Source: CAD feature listing. Evaluate the final solid. Frame: model axes, mm. Give positions to 0.01 mm unless a question says otherwise; leave off trailing zeros. Return JSON: item names as keys, results as strings.
from build123d import *

# Parameters (mm, degrees)
SWEEP1_PROFILE_R     = 13.49375
CUT_SWEEP1_PROFILE_R = 9.525


with BuildPart() as part:
    # Sweep1: sweep along a curve in space
    with BuildLine() as sweep1_path:
        Line((1.507056985, -46.735868675, -12.121766428), (-2.89884077, -28.462007596, -9.030396792))
        add(Edge.make_bspline(
            [(-2.89884077, -28.462007596, -9.030396792), (-12.733389263, 12.327675443, -2.130049512), (3.694377524, 97.398918076, 17.871222686), (67.313961037, 102.150301712, -7.831655808)],
            knots=[0, 0, 0, 0, 1, 1, 1, 1], degree=3))
        Line((67.313961037, 102.150301712, -7.831655808), (90.808311358, 103.904960663, -17.323582638))
    # Sweep1 profile (on start of the path) → Sweep1 (sweep)
    with BuildSketch(Plane(origin=(1.507056985, -46.735868675, -12.121766428), x_dir=(0.9721432612515077, 0.23438745615600456, 0), z_dir=(-0.23128072205980613, 0.959257799436907, 0.16227662130743767))):
        Circle(SWEEP1_PROFILE_R)
    sweep(path=sweep1_path.line, is_frenet=True)

    # Cut-Sweep1: sweep along a curve in space
    with BuildLine() as cut_sweep1_path:
        Line((1.507056985, -46.735868675, -12.121766428), (-2.89884077, -28.462007596, -9.030396792))
        add(Edge.make_bspline(
            [(-2.89884077, -28.462007596, -9.030396792), (-12.733389263, 12.327675443, -2.130049512), (3.694377524, 97.398918076, 17.871222686), (67.313961037, 102.150301712, -7.831655808)],
            knots=[0, 0, 0, 0, 1, 1, 1, 1], degree=3))
        Line((67.313961037, 102.150301712, -7.831655808), (90.808311358, 103.904960663, -17.323582638))
    # Cut-Sweep1 profile (on start of the path) → Cut-Sweep1 (sweep, cut)
    with BuildSketch(Plane(origin=(1.507056985, -46.735868675, -12.121766428), x_dir=(0.9721432612515077, 0.23438745615600456, 0), z_dir=(-0.23128072205980613, 0.959257799436907, 0.16227662130743767))):
        Circle(CUT_SWEEP1_PROFILE_R)
    sweep(path=cut_sweep1_path.line, mode=Mode.SUBTRACT)


solid = part.part
1. Draft query along X for faces 1 (the face through (-1.941, -46.034, -21.185)), 2 (the face through (11.587, -35.365, -5.455)), 3 (the face through (-10, -39.6, -11)). Return one class per face: pulls with the +X half, pulls with the -X half, needs draft (parallel to the pull), parting line crosses it, or undercut.
Evaluation:
{"face 1": "pulls with the +X half", "face 2": "parting line crosses it", "face 3": "undercut"}
2. First-contact query: pin 1 (3 mm diameter, centred on x = 75.5, z = -3, fed in from +Y); pin 2 (1.5 mm diameter, centred on x = 53.5, y = 87.5, fed in from +Z); pin 3 (4 mm diameter, centred on y = 68.5, z = 11, fed in from -X). Flat tips, straight axial feed; report the tip coordinate or a pass-through.
Evaluation:
{"pin 1": "stops at y = 114.65", "pin 2": "stops at z = 7.02", "pin 3": "stops at x = -1.43"}
3. Ray query, probe 1 along Y at (x, z) = (35, -1); probe 2 along Y at (x, z) = (40, -7.5); probe 3 along X at (y, z) = (84.5, 11). Return the intervals inside material, ascending.
Evaluation:
{"probe 1": "y = 74.78 to 80.35, 101.8 to 106.52", "probe 2": "y = 83.17 to 90.43, 99.94 to 106.74", "probe 3": "x = 10.74 to 17.27, 35.45 to 43.5"}
